Work out the finished part from the listing and answer in its coordinate system (mm). A direction names the side the tool comes from. Give positions to 0.01 mm unless a question says otherwise; leave off trailing zeros. Order: outer loops, then holes, each group sorted by start corner. A loop starts at its lowest first (then second) coordinate and runs counter-clockwise, first axis right, second up.
```python
from build123d import *

# Parameters (mm, degrees)
S01_CORD_EYE_LINER_R                 = 2
S01_CORD_EYE_LINER_R_2               = 1.1
F_01_CORD_EYE_LINER_DEPTH            = 11
F_02_START                           = -0.45
S02_SWAGED_REAR_RETENTION_LIP_R      = 2.62
S02_SWAGED_REAR_RETENTION_LIP_R_2    = 1.1
F_02_SWAGED_REAR_RETENTION_LIP_DEPTH = 0.45
F_03_START                           = 11
S03_MOUTH_FLANGE_R                   = 3.1
S03_MOUTH_FLANGE_R_2                 = 1.4
F_03_MOUTH_FLANGE_DEPTH              = 1
F_04_START                           = 10.2
S04_INLET_RELIEF_R                   = 1.25
F_04_INLET_RELIEF_DEPTH              = 0.9


with BuildPart() as part:
    # S01 - Cord eye liner → 01 - Cord eye liner (new body)
    with BuildSketch(Plane.XY):
        Circle(S01_CORD_EYE_LINER_R)
        Circle(S01_CORD_EYE_LINER_R_2, mode=Mode.SUBTRACT)
    extrude(amount=F_01_CORD_EYE_LINER_DEPTH)

    # S02 - Swaged rear retention lip → 02 - Swaged rear retention lip (add)
    with BuildSketch(Plane.XY.offset(F_02_START)):
        Circle(S02_SWAGED_REAR_RETENTION_LIP_R)
        Circle(S02_SWAGED_REAR_RETENTION_LIP_R_2, mode=Mode.SUBTRACT)
    extrude(amount=F_02_SWAGED_REAR_RETENTION_LIP_DEPTH)

    # S03 - Mouth flange → 03 - Mouth flange (add)
    with BuildSketch(Plane.XY.offset(F_03_START)):
        Circle(S03_MOUTH_FLANGE_R)
        Circle(S03_MOUTH_FLANGE_R_2, mode=Mode.SUBTRACT)
    extrude(amount=F_03_MOUTH_FLANGE_DEPTH)

    # S04 - Inlet relief → 04 - Inlet relief (cut)
    with BuildSketch(Plane.XY.offset(F_04_START)):
        Circle(S04_INLET_RELIEF_R)
    extrude(amount=F_04_INLET_RELIEF_DEPTH, mode=Mode.SUBTRACT)


solid = part.part
```
1. Given P1, Ø2.5, axis at x = 0, y = 0, coming from the -Z side; P2, Ø1.5, axis at y = -1, z = 1, coming from the +X side; P3, Ø3, axis at x = -1, z = 9, coming from the -Y side; P4, Ø1, axis at x = 1, z = 4, coming from the -Y side, each flat-ended and moving along its own axis, determine where each tip first touches the part or whether it passes through.
Findings below:
P1: stops at z = -0.45
P2: stops at x = 1.98
P3: stops at y = -2
P4: stops at y = -1.94
2. The part is cut by section C-C (z = 8). Write down the section's boundary in (x, y).
Findings below:
outline: circle Ø4 at (0, 0); hole circle Ø2.2 at (0, 0)
3. The mould has two halves that part along Z. Classify faces 5 (the face through (-1, -2, 0)), 6 (the face through (2, -1, 11)), 7 (the face through (1.05, 0.33, 4.8)), 8 (the face through (1, -1, -0.45)): pulls with the +Z half, pulls with the -Z half, needs draft (parallel to the pull), parting line crosses it, or undercut.
Findings below:
face 5: undercut
face 6: undercut
face 7: needs draft
face 8: pulls with the -Z half
4. Straight lines are drawn through the part: probe 1 along Z at (x, y) = (-1, 2); probe 2 along Y at (x, z) = (0, 10.5); probe 3 along Y at (x, z) = (0, 11.3). For each, find the intervals that lie inside material, in ascending order.
Findings below:
probe 1: z = -0.45 to 0, 11 to 12
probe 2: y = -2 to -1.25, 1.25 to 2
probe 3: y = -3.1 to -1.4, 1.4 to 3.1
5. The part is cut by section D-D (x = -1.75). Write down the section's boundary in (y, z), then the cut area to 3 significant figures.
Findings below:
outline: (-2.56, 11) - (-0.97, 11) - (-0.97, 0) - (-1.95, 0) - (-1.95, -0.45) - (1.95, -0.45) - (1.95, 0) - (0.97, 0) - (0.97, 11) - (2.56, 11) - (2.56, 12) - (-2.56, 12) - close
area: 28.2 mm2
6. The part is cut by section A-A (y = 0). Write down the section's boundary in (x, z).
Findings below:
outline: (-3.1, 11) - (-2, 11) - (-2, 0) - (-2.62, 0) - (-2.62, -0.45) - (-1.1, -0.45) - (-1.1, 10.2) - (-1.25, 10.2) - (-1.25, 11) - (-1.4, 11) - (-1.4, 12) - (-3.1, 12) - close; (1.1, -0.45) - (2.62, -0.45) - (2.62, 0) - (2, 0) - (2, 11) - (3.1, 11) - (3.1, 12) - (1.4, 12) - (1.4, 11) - (1.25, 11) - (1.25, 10.2) - (1.1, 10.2) - close
7. Which of the six approach directions +Z, -Z, +X, -X, +Y, -Y give full straight-line access (tool end or side, diameter ignored) to faces 1 (the face through (-0.341, 2.598, -0.228)), 2 (the face through (1.43, -2.75, 11.49)), 3 (the face through (0, -2, 5)), 4 (the face through (-1.4, 0.06, 11.49))?
Findings below:
face 1: -Z
face 2: +Z, -Z
face 3: none
face 4: +Z
